Read the model definition and answer for the solid it produces. Units are mm, in the model's axes. Coordinates: 2 decimals unless noted, no trailing zeros. Write each loop counter-clockwise with the first axis right and the second up, starting at its lowest first coordinate (ties: lowest second). Pieces come first, ordered by that corner, then holes. Notation, with made-up numbers: (42.5, -38.75) - (94.5, -38.75) arc R24 cw to (94.5, -21.75) - close; hole circle Ø7 at (66.25, -37.5). An arc over 180 degrees is marked (long way). Return JSON: item names as keys, results as strings.
```python
from build123d import *

# Parameters (mm, degrees)
SKETCH1_W           = 163
SKETCH1_H           = 210.5
BOSS_EXTRUDE1_DEPTH = 3
SKETCH2_W           = 2.7
SKETCH2_H           = 10
CUT_EXTRUDE1_DEPTH  = 3
SKETCH3_W           = 86
SKETCH3_H           = 74
CUT_EXTRUDE2_DEPTH  = 1.5
CUT_EXTRUDE3_REACH  = 3.5
SKETCH4_W           = 25
SKETCH4_H           = 3
CUT_EXTRUDE5_REACH  = 5
SKETCH5_R           = 1.5
SKETCH5_R_2         = 6.5


with BuildPart() as part:
    # Sketch1 → Boss-Extrude1 (new body)
    with BuildSketch(Plane.XY):
        Rectangle(SKETCH1_W, SKETCH1_H)
    extrude(amount=BOSS_EXTRUDE1_DEPTH)

    # Sketch2 → Cut-Extrude1 (cut)
    with BuildSketch(Plane.XY.offset(3)):
        with Locations((-76.65, -85.25)):
            Rectangle(SKETCH2_W, SKETCH2_H)
        with Locations((-76.65, 84.15)):
            Rectangle(SKETCH2_W, SKETCH2_H)
    cut_extrude1 = extrude(amount=-CUT_EXTRUDE1_DEPTH, mode=Mode.SUBTRACT)

    # Mirror3: Cut-Extrude1 across plane
    add(cut_extrude1.mirror(Plane(origin=(0, 0, 0), x_dir=(0, 0, 1), z_dir=(1, 0, 0))), mode=Mode.SUBTRACT)

    # Sketch3 → Cut-Extrude2 (cut)
    with BuildSketch(Plane.XY.offset(3)):
        with Locations((26.5, 46.5)):
            Rectangle(SKETCH3_W, SKETCH3_H)
    extrude(amount=-CUT_EXTRUDE2_DEPTH, mode=Mode.SUBTRACT)

    # Sketch4 → Cut-Extrude3 (cut, up to next)
    with BuildSketch(Plane.XY.offset(1.5), mode=Mode.PRIVATE) as cut_extrude3_sk1:
        with Locations((0, 82)):
            Rectangle(SKETCH4_W, SKETCH4_H)
    cut_extrude3_tool1 = extrude(cut_extrude3_sk1.sketch, amount=-CUT_EXTRUDE3_REACH, mode=Mode.PRIVATE) & part.part
    add(cut_extrude3_tool1.solids().sort_by_distance((0, 82, 1.5))[0], mode=Mode.SUBTRACT)

    # Sketch5 → Cut-Extrude5 (cut, up to next)
    with BuildSketch(Plane.XY.offset(3), mode=Mode.PRIVATE) as cut_extrude5_sk1:
        with Locations((-46.5, 75.25)):
            Circle(SKETCH5_R)
    cut_extrude5_tool1 = extrude(cut_extrude5_sk1.sketch, amount=-CUT_EXTRUDE5_REACH, mode=Mode.PRIVATE) & part.part
    add(cut_extrude5_tool1.solids().sort_by_distance((-46.5, 75.25, 3))[0], mode=Mode.SUBTRACT)
    # Sketch5 → Cut-Extrude5 (cut, up to next)
    with BuildSketch(Plane.XY.offset(3), mode=Mode.PRIVATE) as cut_extrude5_sk2:
        with Locations((-46.5, 55.25)):
            Circle(SKETCH5_R)
    cut_extrude5_tool2 = extrude(cut_extrude5_sk2.sketch, amount=-CUT_EXTRUDE5_REACH, mode=Mode.PRIVATE) & part.part
    add(cut_extrude5_tool2.solids().sort_by_distance((-46.5, 55.25, 3))[0], mode=Mode.SUBTRACT)
    # Sketch5 → Cut-Extrude5 (cut, up to next)
    with BuildSketch(Plane.XY.offset(3), mode=Mode.PRIVATE) as cut_extrude5_sk3:
        with Locations((-46.5, 35.25)):
            Circle(SKETCH5_R)
    cut_extrude5_tool3 = extrude(cut_extrude5_sk3.sketch, amount=-CUT_EXTRUDE5_REACH, mode=Mode.PRIVATE) & part.part
    add(cut_extrude5_tool3.solids().sort_by_distance((-46.5, 35.25, 3))[0], mode=Mode.SUBTRACT)
    # Sketch5 → Cut-Extrude5 (cut, up to next)
    with BuildSketch(Plane.XY.offset(3), mode=Mode.PRIVATE) as cut_extrude5_sk4:
        with Locations((-46.5, 15.25)):
            Circle(SKETCH5_R_2)
    cut_extrude5_tool4 = extrude(cut_extrude5_sk4.sketch, amount=-CUT_EXTRUDE5_REACH, mode=Mode.PRIVATE) & part.part
    add(cut_extrude5_tool4.solids().sort_by_distance((-46.5, 15.25, 3))[0], mode=Mode.SUBTRACT)


solid = part.part
```
(1) A cutting plane is placed at D-D (x = 64). Determine the outline of the cut face in (y, z).
Answer:
{"outline": "(-105.25, 0) - (105.25, 0) - (105.25, 3) - (83.5, 3) - (83.5, 1.5) - (9.5, 1.5) - (9.5, 3) - (-105.25, 3) - close"}
(2) Determine the mould class of faces 1 (the face through (-52.994, 15.536, 1.521)), 2 (the face through (-1, 1, 0)), 3 (the face through (26, 47, 1.5)) for opening direction X: +X half, -X half, draft (parallel to the pull), parting line (faces both ways), or undercut.
Answer:
{"face 1": "undercut", "face 2": "draft", "face 3": "undercut"}
(3) Flat-ended cylindrical pins translate along their axes: P1, Ø8, axis at x = -27.5, y = -81, coming from the -Z side; P2, Ø2.5, axis at x = -46.5, y = 55.25, coming from the -Z side. Find the tip coordinate at first contact, or state that the pin passes through.
Answer:
{"P1": "z = 0", "P2": "through"}
(4) A cutting plane is placed at B-B (z = 2.35). State how many separate pieces and enclosed holes the cut face has, and give its area (3 significant figures).
Answer:
{"separate pieces": "1", "enclosed holes": "9", "area": "27,700 mm²"}
(5) A cutting plane is placed at C-C (y = 40.5). Determine the outline of the cut face in (x, z).
Answer:
{"outline": "(-81.5, 0) - (81.5, 0) - (81.5, 3) - (69.5, 3) - (69.5, 1.5) - (-16.5, 1.5) - (-16.5, 3) - (-81.5, 3) - close"}
(6) Straight lines are drawn through the part: line 1 (Y direction, x = -46.5, z = 1.65); line 2 (X direction, y = 75.25, z = 2); line 3 (Y direction, x = 22, z = 1.75). For each, find the intervals that lie inside material, in ascending order. Write a range as from..to.
Answer:
{"line 1": "-105.25..8.75, 21.75..33.75, 36.75..53.75, 56.75..73.75, 76.75..105.25", "line 2": "-81.5..-48, -45..-16.5, 69.5..81.5", "line 3": "-105.25..9.5, 83.5..105.25"}
(7) A cutting plane is placed at A-A (y = 15.25). Determine the outline of the cut face in (x, z), and give its area (3 significant figures).
Answer:
{"outline": "(-81.5, 0) - (-53, 0) - (-53, 3) - (-81.5, 3) - close; (-40, 0) - (81.5, 0) - (81.5, 3) - (69.5, 3) - (69.5, 1.5) - (-16.5, 1.5) - (-16.5, 3) - (-40, 3) - close", "area": "321 mm²"}
